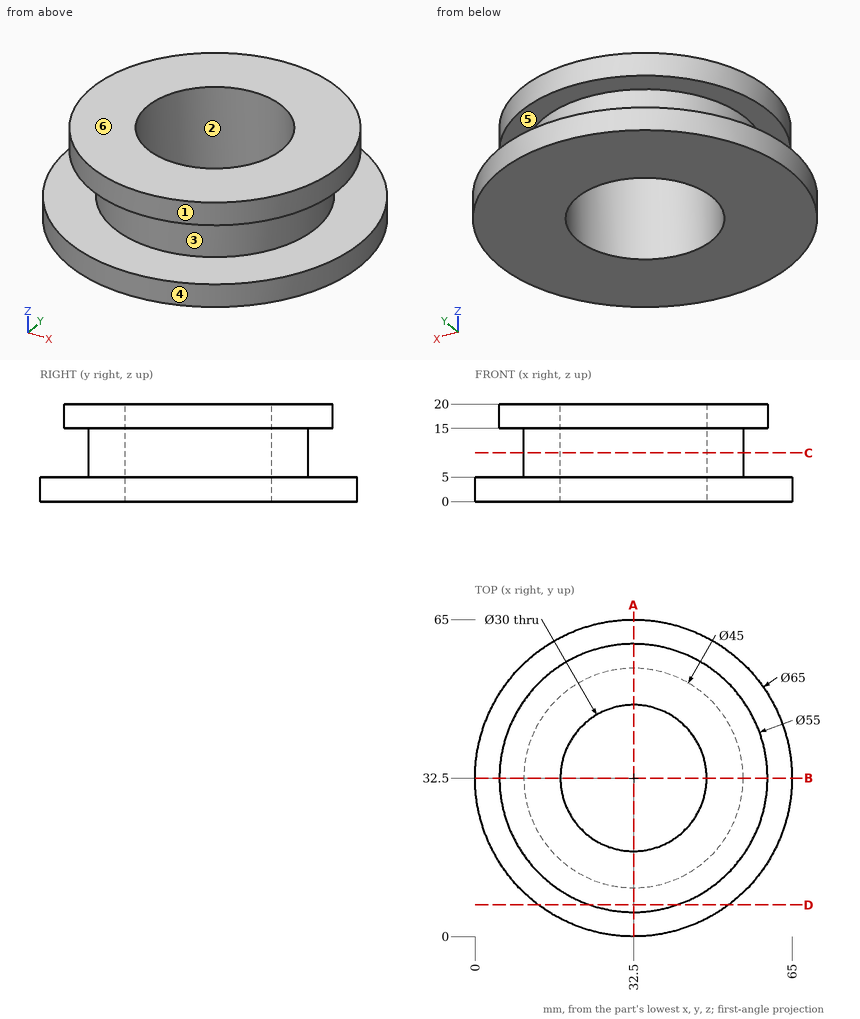
Geometry: see drawing. Coordinates: mm, zero at the bounding-box minimum. A direction names the side the tool comes from. Give positions to 0.01 mm unless a question says otherwise; leave off trailing zeros. Write each loop counter-clockwise with the first axis right and the second up, starting at its lowest first coordinate (ties: lowest second). Pieces come first, ordered by that corner, then holes. Notation, with made-up numbers: M 67,-1.75 L 126,-1.75 A30 cw 126,28.25 Z; hole C 34,3.5 d9. An arc over 180 degrees is marked long. Return JSON: item names as keys, results as strings. Group by question number.
1) Set-up query: the marked faces 1, 2 and 3. Return all of +Z, -Z, +X, -X, +Y, -Y with unobstructed straight access to the full face (end or side cutting, diameter ignored); none if empty.
2) Draft query along Z for the marked faces 4, 5 and 6. Return one class per face: released by +Z, released by -Z, zero draft, split by the parting line, or undercut.
3) Cut plane C-C, the plane z = 10. Output: boundary loops of the cut face in (x, y), then the cut area to 3 significant figures.
4) Cut plane D-D, the plane y = 6.5. Output: boundary loops of the cut face in (x, z), then the cut area to 3 significant figures.
5) Cut plane A-A, the plane x = 32.5. Output: boundary loops of the cut face in (y, z), then the cut area to 3 significant figures.
6) Ray query, L1, parallel to Y at x = 32.5, z = 4; L2, parallel to Y at x = 32.5, z = 12; L3, parallel to Z at x = 54.5, y = 27.5. Return the intervals inside material, ascending.
7) First-contact query: pin 1 Ø5 at (x, y) = (21.5, 25.5) entering from +Z; pin 2 Ø6 at (x, z) = (12, 14) entering from +Y; pin 3 Ø4 at (y, z) = (47.5, 18) entering from -X; pin 4 Ø4 at (y, z) = (49, 10) entering from +X. Flat tips, straight axial feed; report the tip coordinate or a pass-through.
Data:
{
 "1": {"face 1": "+Z", "face 2": "+Z, -Z", "face 3": "none"},
 "2": {"face 4": "zero draft", "face 5": "undercut", "face 6": "released by +Z"},
 "3": {"outline": "C 32.5,32.5 d45; hole C 32.5,32.5 d30", "area": "884 mm²"},
 "4": {"outline": "M 13,0 L 52,0 L 52,5 L 13,5 Z; M 23.54,15 L 41.46,15 L 41.46,20 L 23.54,20 Z", "area": "285 mm²"},
 "5": {"outline": "M 0,0 L 17.5,0 L 17.5,20 L 5,20 L 5,15 L 10,15 L 10,5 L 0,5 Z; M 47.5,0 L 65,0 L 65,5 L 55,5 L 55,15 L 60,15 L 60,20 L 47.5,20 Z", "area": "450 mm²"},
 "6": {"L1": "y = 0 to 17.5, 47.5 to 65", "L2": "y = 10 to 17.5, 47.5 to 55", "L3": "z = 0 to 5, 15 to 20"},
 "7": {"pin 1": "stops at z = 20", "pin 2": "stops at y = 53.57", "pin 3": "stops at x = 8.27", "pin 4": "stops at x = 49.7"}
}
